Part print with two shaded views. Sizes in mm from the minimum x, y, z corner. Coordinates: 2 decimals unless noted, no trailing zeros. Write each loop counter-clockwise with the first axis right and the second up, starting at its lowest first coordinate (ties: lowest second). Pieces come first, ordered by that corner, then holes. Notation, with made-up numbers: (29, 55) - (38, 55) arc R20 cw to (38, 89) - close; hole circle Ø3 at (81, 57). An arc over 180 degrees is marked (long way). One line per question, with ' | ' between items. Start each with the question number.
1. Band-saw the part on D-D, the plane z = 30.5. Write the cut outline in (x, y), then the cut area to 3 significant figures.
2. Probe line 1 (Y direction, x = 0.95, z = 119); line 2 (Z direction, x = 1.8, y = 20); line 3 (Y direction, x = 0.8, z = 95). List the from-to ranges inside material, lowest first.
3. Band-saw the part on A-A, the plane y = 22. Write the cut outline in (x, z), then the cut area to 3 significant figures.
4. Flat gauge pins, fed straight in: P1, Ø1.5, axis at x = 1, z = 164, coming from the +Y side; P2, Ø0.9, axis at x = 1, z = 3, coming from the -Y side; P3, Ø1.5, axis at x = 1, y = 141.5, coming from the -Z side. Where does each tip first touch, or does it go through?
5. Band-saw the part on C-C, the plane z = 58.5. Write the cut outline in (x, y).
6. Band-saw the part on B-B, the plane x = 2.3. Write the cut outline in (y, z), then the cut area to 3 significant figures.
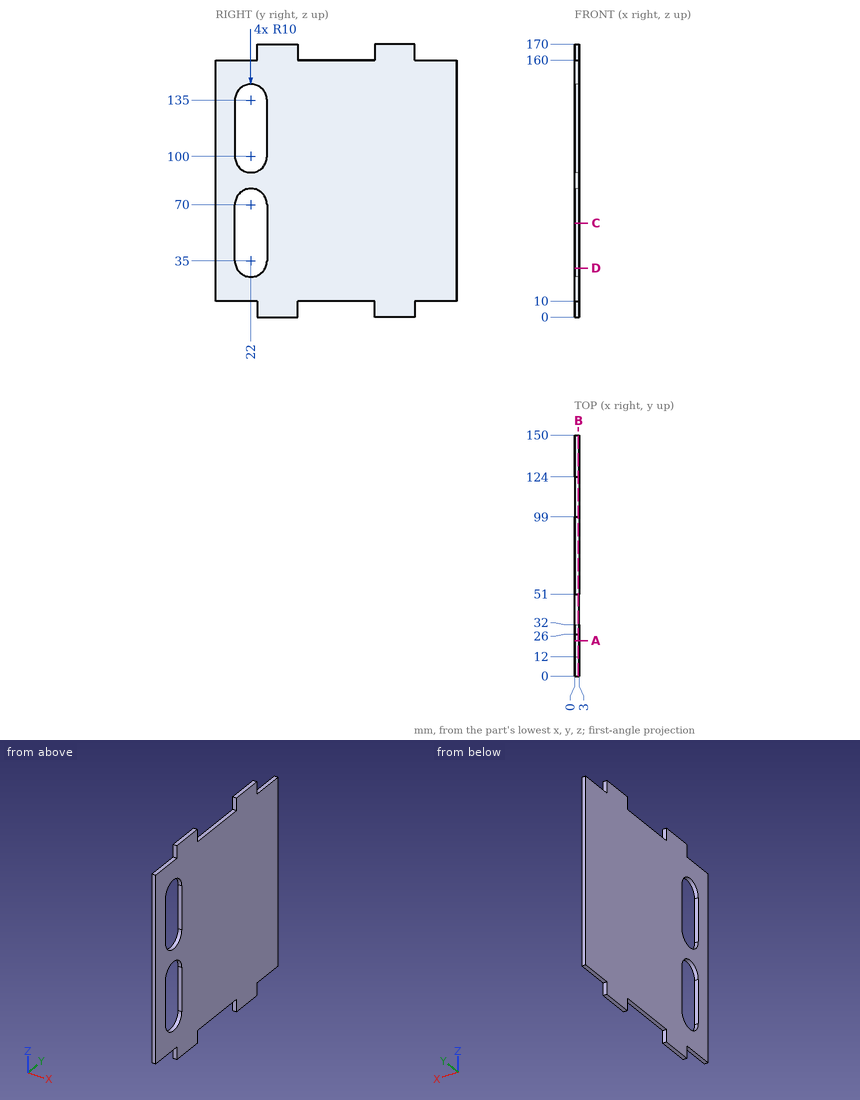
Filled in:
1) outline: (0, 0) - (3, 0) - (3, 13.07) - (0, 13.07) - close; (0, 30.93) - (3, 30.93) - (3, 150) - (0, 150) - close | area: 396 mm²
2) line 1: y = 0 to 12, 32 to 150 | line 2: z = 10 to 25.2, 79.8 to 90.2, 144.8 to 160 | line 3: y = 0 to 13.34, 30.66 to 150
3) outline: (0, 10) - (3, 10) - (3, 25) - (0, 25) - close; (0, 80) - (3, 80) - (3, 90) - (0, 90) - close; (0, 145) - (3, 145) - (3, 160) - (0, 160) - close | area: 120 mm²
4) P1: stops at y = 124 | P2: stops at y = 26 | P3: stops at z = 10
5) outline: (0, 0) - (3, 0) - (3, 12) - (0, 12) - close; (0, 32) - (3, 32) - (3, 150) - (0, 150) - close
6) outline: (0, 10) - (26, 10) - (26, 0) - (51, 0) - (51, 10) - (99, 10) - (99, 0) - (124, 0) - (124, 10) - (150, 10) - (150, 160) - (124, 160) - (124, 170) - (99, 170) - (99, 160) - (51, 160) - (51, 170) - (26, 170) - (26, 160) - (0, 160) - close; hole (12, 35) arc R10 ccw to (32, 35) - (32, 70) arc R10 ccw to (12, 70) - close; hole (12, 100) arc R10 ccw to (32, 100) - (32, 135) arc R10 ccw to (12, 135) - close | area: 21,500 mm²
